Geometry check sheet. Reference: drawing and pictorial views, mm from the part's lowest x, y, z. A direction names the side the tool comes from. Coordinates: 2 decimals unless noted, no trailing zeros. Loops run counter-clockwise (first coordinate to the right, second up) from the corner with the lowest first, then second, coordinate; pieces in that order, holes last. Notation, with made-up numbers: M 53,59.5 L 100,59.5 A20 ccw 100,87.5 Z; hole C 30.25,57.5 d8. An arc over 180 degrees is marked long. Write item = value, one per line. Start each with the question number.
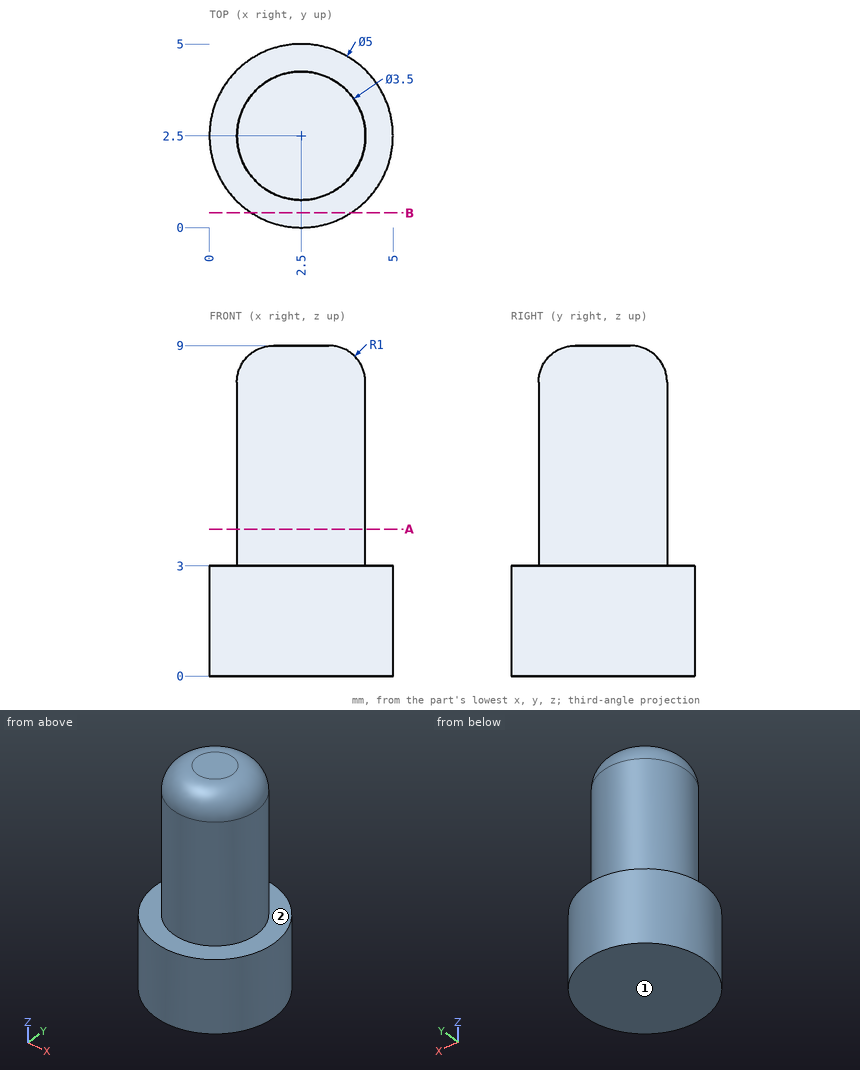
Q1. Gauge pin test, flat ends, axial feed: pin 1 (1 mm diameter, centred on x = 1.5, z = 7.5, fed in from -Y); pin 2 (1.5 mm diameter, centred on y = 3.5, z = 7, fed in from -X); pin 3 (1.5 mm diameter, centred on y = 4, z = 2.5, fed in from -X). Record the tip position at first contact, or that the pin passes through.
Q2. Scan lines: L1, parallel to Z at x = 0.85, y = 3.45; L2, parallel to X at y = 2.5, z = 5.5. Record each from-to range of solid material in increasing order. Write a range as [from, to].
Q3. Sectioned sample at A-A on z = 4. Record the cut outline in (x, y).
Q4. Sectioned sample at B-B on y = 0.4. Record the cut outline in (x, z).
Q5. Set-up check for the marked faces 1 and 2: record each of +Z, -Z, +X, -X, +Y, -Y from which the full face is reachable in a straight line by a thin tool's end or side.
Solutions:
q1.pin_1 = 0.82
q1.pin_2 = 0.77
q1.pin_3 = 0.12
q2.L1 = [0, 3]
q2.L2 = [0.75, 4.25]
q3.outline = C 2.5,2.5 d3.5
q4.outline = M 1.14,0 L 3.86,0 L 3.86,3 L 1.14,3 Z
q5.face_1 = -Z, +X, -X, +Y, -Y
q5.face_2 = +Z
